from build123d import *

# Parameters (mm, degrees)
SKETCH1_R           = 14.2
SKETCH1_R_2         = 12.6
BOSS_EXTRUDE1_DEPTH = 16
BOSS_EXTRUDE2_DEPTH = 3.2
SKETCH3_R           = 1.55
CUT_EXTRUDE1_DEPTH  = 10
FILLET1_R           = 2
SKETCH4_R           = 12.6
SKETCH4_R_2         = 3.8
BOSS_EXTRUDE3_DEPTH = 0.8


with BuildPart() as part:
    # Sketch1 → Boss-Extrude1 (new body)
    with BuildSketch(Plane(origin=(0, 0, 0), x_dir=(1, 0, 0), z_dir=(0, 1, 0))):
        with Locations(Location((0, 0, 0), (0, 0, 270))):
            Circle(SKETCH1_R)
        with Locations(Location((0, 0, 0), (0, 0, 270))):
            Circle(SKETCH1_R_2, mode=Mode.SUBTRACT)
    extrude(amount=BOSS_EXTRUDE1_DEPTH)

    # Sketch2 → Boss-Extrude2 (add)
    with BuildSketch(Plane(origin=(0, 0, 0), x_dir=(-1, 0, 0), z_dir=(0, -1, 0))):
        with BuildLine():
            Line((7.592101158, -12), (22.4, -12))
            Line((22.4, -12), (22.4, 12))
            Line((22.4, 12), (7.592101158, 12))
            ThreePointArc((7.592101158, 12), (12.438806945, 6.8495315), (14.2, 0))
            ThreePointArc((14.2, 0), (12.438806945, -6.8495315), (7.592101158, -12))
        make_face()
    extrude(amount=-BOSS_EXTRUDE2_DEPTH)

    # Sketch3 → Cut-Extrude1 (cut)
    with BuildSketch(Plane(origin=(0, 0, 0), x_dir=(-1, 0, 0), z_dir=(0, -1, 0))):
        with Locations(Location((18.4, 6, 0), (0, 0, 90))):
            Circle(SKETCH3_R)
        with Locations(Location((18.4, -6, 0), (0, 0, 90))):
            Circle(SKETCH3_R)
    extrude(amount=-CUT_EXTRUDE1_DEPTH, mode=Mode.SUBTRACT)

    # Fillet1
    fillet1_edges = [part.edges().sort_by_distance(p)[0] for p in [
        (-14.2, 3.2, 0),
    ]]
    fillet(fillet1_edges, radius=FILLET1_R)

    # Sketch4 → Boss-Extrude3 (add)
    with BuildSketch(Plane(origin=(0, 0, 0), x_dir=(-1, 0, 0), z_dir=(0, -1, 0))):
        with Locations(Location((0, 0, 0), (0, 0, 90))):
            Circle(SKETCH4_R)
        with Locations(Location((0, 0, 0), (0, 0, 90))):
            Circle(SKETCH4_R_2, mode=Mode.SUBTRACT)
    extrude(amount=-BOSS_EXTRUDE3_DEPTH)


solid = part.part
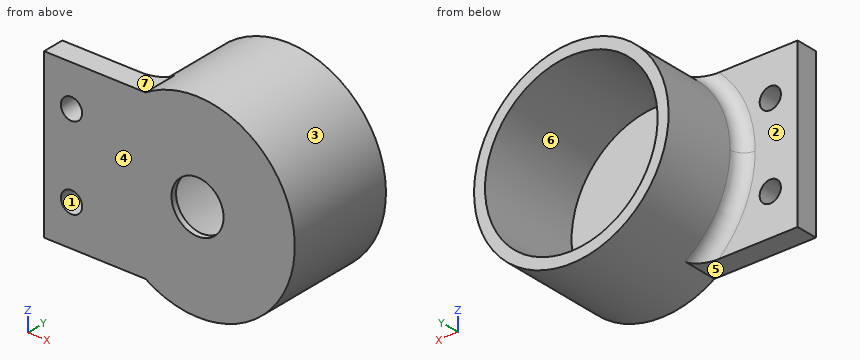
Geometry: final body of the model. Coordinates: model frame, mm. Face numbers are marked on the shaded views. A direction names the side the tool comes from. Coordinates: 2 decimals unless noted, no trailing zeros. Loops run counter-clockwise (first coordinate to the right, second up) from the corner with the lowest first, then second, coordinate; pieces in that order, holes last. Notation, with made-up numbers: (41.5, 33) - (75.5, 33) arc R30 ccw to (75.5, 61) - close; hole circle Ø2 at (36, 46). An arc over 180 degrees is marked (long way). Put each result on its own line as item: value. Start each with the question number.
Q1. Cut plane B-B, the plane x = -18.4. Return loops of the section in (y, z), and give its area (3 significant figures).
Q2. Set-up query: the marked faces 4, 5, 6 and 7. Return all of +Z, -Z, +X, -X, +Y, -Y with unobstructed straight access to the full face (end or side cutting, diameter ignored); none if empty.
Q3. Pin query (flat end, axial travel): pin 1 Ø3 at (x, y) = (-6, 4) entering from +Z; pin 2 Ø3.5 at (x, z) = (-18, 3.5) entering from +Y; pin 3 Ø10 at (x, z) = (0, 0) entering from +Y; pin 4 Ø5 at (x, y) = (-1.5, 6) entering from -Z. Return the tip coordinate at first contact, or that it passes through.
Q4. Cut plane C-C, the plane y = 2.25. Return loops of the section in (x, z).
Q5. Pull-direction query (Z, two-part tool) for the marked faces 1, 2 and 3; classes: released by +Z, released by -Z, zero draft, split by the parting line, or undercut.
Q6. Cut plane A-A, the plane x = 0. Return loops of the section in (y, z), and give its area (3 significant figures).
Q7. Cut plane D-D, the plane y = 9.25. Return loops of the section in (x, z), and give its area (3 significant figures).
Q8. Line query: line 1 (X direction, y = 0.45, z = 0); line 2 (X direction, y = 12.5, z = 0.25); line 3 (X direction, y = 2.1, z = 6). Output: solid intervals per line, ascending.
Filled sheet:
1. outline: (0, -12) - (3.2, -12) - (3.2, -7.55) - (0, -7.55) - close; (0, -4.45) - (3.2, -4.45) - (3.2, 4.45) - (0, 4.45) - close; (0, 7.55) - (3.2, 7.55) - (3.2, 12) - (0, 12) - close
1. area: 57.0 mm²
2. face 4: +Z, -Z, +X, -X, -Y
2. face 5: -Z, -X, +Y, -Y
2. face 6: +Y
2. face 7: +Z, -X, +Y, -Y
3. pin 1: z = 13.47
3. pin 2: y = 3.2
3. pin 3: y = 0.8
3. pin 4: z = -14.2
4. outline: (-22.4, -12) - (-7.59, -12) arc R14.2 ccw (long way) to (-7.59, 12) - (-22.4, 12) - close; hole circle Ø3.1 at (-18.4, -6); hole circle Ø3.1 at (-18.4, 6); hole circle Ø25.2 at (0, 0)
5. face 1: undercut
5. face 2: zero draft
5. face 3: split by the parting line
6. outline: (0, -14.2) - (16, -14.2) - (16, -12.6) - (0.8, -12.6) - (0.8, -3.8) - (0, -3.8) - close; (0, 3.8) - (0.8, 3.8) - (0.8, 12.6) - (16, 12.6) - (16, 14.2) - (0, 14.2) - close
6. area: 65.3 mm²
7. outline: circle Ø28.4 at (0, 0); hole circle Ø25.2 at (0, 0)
7. area: 135 mm²
8. line 1: -22.4 to -3.8, 3.8 to 14.2
8. line 2: -14.2 to -12.6, 12.6 to 14.2
8. line 3: -22.4 to -19.95, -16.85 to -11.08, 11.08 to 12.87
